Input: part model. Units: mm. Frame: model coordinates. A direction names the side the tool comes from. Round coordinates to 2 decimals unless told otherwise and drop trailing zeros. Order: outer loops, then holes, each group sorted by start corner. A loop starts at its lowest first (then second) coordinate and runs counter-clockwise, first axis right, second up. Notation, with made-up numbers: (64.5, 51.5) - (119.5, 51.5) arc R21 ccw to (119.5, 79.5) - close; hole circle Ø5 at (72.5, 6.5). An arc over 180 degrees is marked (long way). One line per item, written item: value. Start each with the question number.
from build123d import *

# Parameters (mm, degrees)
F0_R      = 15
F1_DEPTH  = 28
F1_FACE_R = 15
F2_DEPTH  = 25.4
F3_R      = 15
F4_DEPTH  = 28


with BuildPart() as f1:
    # F0 (on Front) → F1 (new body)
    with BuildSketch(Plane.XZ):
        Circle(F0_R)
    extrude(amount=F1_DEPTH)

    # F1_face (on face) → F2 (join)
    with BuildSketch(Plane(origin=(0, 0, 0), x_dir=(1, 0, 0), z_dir=(0, 1, 0))):
        Circle(F1_FACE_R)
    extrude(amount=F2_DEPTH)

    # F3 (on Right) → F4 (join)
    with BuildSketch(Plane.YZ):
        Circle(F3_R)
    extrude(amount=F4_DEPTH)


solid = f1.part
1. Line query: line 1 (X direction, y = -19, z = -4.5); line 2 (X direction, y = -7.5, z = 3.75); line 3 (Z direction, x = 3.5, y = -13). Output: solid intervals per line, ascending. Write a range as from..to.
2. Set-up query: faces 1 (the face through (-14.985, -1.674, -0.66)), 2 (the face through (28, 0, 0)), 3 (the face through (16.915, -3.252, -14.643)). Return all of +Z, -Z, +X, -X, +Y, -Y with unobstructed straight access to the full face (end or side cutting, diameter ignored); none if empty.
3. Section A-A (z = 9). Return the cut outline in (x, y), then the cut area to 3 significant figures.
4. Pin query (flat end, axial travel): pin 1 (1.5 mm diameter, centred on x = 15, z = 5, fed in from -Y); pin 2 (6 mm diameter, centred on y = -14.5, z = 9.5, fed in from -X); pin 3 (1.5 mm diameter, centred on x = -10, y = 17.5, fed in from +Z). Return the tip coordinate at first contact, or that it passes through.
5. Section B-B (x = 13). Return the cut outline in (y, z), then the cut area to 3 significant figures.
6. Section C-C (y = -20.5). Return the cut outline in (x, z).
7. Section D-D (y = 0). Return the cut outline in (x, z), then the cut area to 3 significant figures.
Solved:
1. line 1: x = -14.31..14.31
1. line 2: x = -14.52..28
1. line 3: z = -14.59..14.59
2. face 1: none
2. face 2: +Z, -Z, +X, +Y, -Y
2. face 3: +X
3. outline: (-12, -28) - (12, -28) - (12, -12) - (28, -12) - (28, 12) - (12, 12) - (12, 25.4) - (-12, 25.4) - close
3. area: 1,670 mm²
4. pin 1: stops at y = -14.39
4. pin 2: stops at x = -13.52
4. pin 3: stops at z = 11.81
5. outline: (-28, -7.48) - (-13, -7.48) arc R15 ccw to (13, -7.48) - (25.4, -7.48) - (25.4, 7.48) - (13, 7.48) arc R15 ccw to (-13, 7.48) - (-28, 7.48) - close
5. area: 1,080 mm²
6. outline: circle Ø30 at (0, 0)
7. outline: (0, -15) - (28, -15) - (28, 15) - (0, 15) arc R15 ccw to start
7. area: 1,190 mm²
